Geometry: final body of the model. Coordinates: model frame, mm. A direction names the side the tool comes from. Give positions to 0.01 mm unless a question says otherwise; leave off trailing zeros. Loops run counter-clockwise (first coordinate to the right, second up) from the corner with the lowest first, then second, coordinate; pieces in that order, holes last. Notation, with made-up numbers: (79, 26) -> (134, 26) arc R10 ccw to (134, 34) -> close; hole circle Ø11 at (9, -26.75). An arc over 180 degrees is marked (long way). One line per question, with ' | ' between items. Start each with the question number.
Item 1: Pin query (flat end, axial travel): P1, Ø1.3, axis at y = -23, z = -18.5, coming from the -X side; P2, Ø2, axis at y = -32, z = -20.5, coming from the +X side (3 decimals); P3, Ø2, axis at y = -32, z = -19.5, coming from the -X side (3 decimals). Return the tip coordinate at first contact, or that it passes through.
Item 2: Set-up query: faces 4 (the flat face through (-11, -27.374, -23)), 5 (the flat face through (-3.625, -32, -22)), 6 (the flat face through (-8.705, -32, -22)), 7 (the flat face through (-6, -30.894, -21)), 8 (the cylindrical face through (18.321, 42.327, 1.878)). Return all of +Z, -Z, +X, -X, +Y, -Y with unobstructed straight access to the full face (end or side cutting, diameter ignored); none if empty.
Item 3: Mould query, pull axis Z, two halves, no side actions, for faces 1 (the cylindrical face through (-0.222, -24.665, -6.643)), 2 (the flat face through (0, 0, 0)), 3 (the cylindrical face through (-28.98, -38.59, 1.88)). Classes: released by +Z, released by -Z, zero draft, split by the parting line, or undercut.
Item 4: Section C-C on x = 14. Return loops of the section in (y, z), then the cut area to 3 significant figures.
Item 5: Section D-D on x = 22. Return loops of the section in (y, z).
Item 6: Material intervals for line 1 along Y through (x, z) = (-5, -6.35); line 2 along X through (y, z) = (-21, 2.5) (3 decimals); line 3 along Y through (x, z) = (3, -1), sorted ascending. Write a range as [from, to].
Item 7: Section A-A on y = 40.5. Return loops of the section in (x, z), then the cut area to 3 significant figures.
Item 8: Section B-B on z = -2. Return loops of the section in (x, y) (3 decimals).
from build123d import *

# Parameters (mm, degrees)
BOSS_EXTRUDE2_DEPTH                 = 3.81
BOSS_EXTRUDE4_DEPTH                 = 31.75
F_8_CLEARANCE_HOLE1_D               = 4.4958
PARACHUTE_SHROUD_HOLE_LOW_PROFILE_D = 3.175
MONOFILAMENT_HOLE_LOW_PROFILE_D     = 3.175
BOSS_EXTRUDE7_REACH                 = 67.656
SKETCH21_W                          = 2.032
SKETCH21_H                          = 5.08
SKETCH21_W_2                        = 5.08
SKETCH21_H_2                        = 2.032
SKETCH22_W                          = 11.064
SKETCH22_H                          = 10.632
BOSS_EXTRUDE8_DEPTH                 = 7.894195
BOSS_EXTRUDE9_REACH                 = 87.468
BOSS_EXTRUDE10_DEPTH                = 5.08
FILLET3_R                           = 0.127


with BuildPart() as part:
    # Sketch3 → Boss-Extrude2 (new body)
    with BuildSketch(Plane.XY):
        with BuildLine():
            Line((-15.875, -38.1), (-15.875, 38.1))
            ThreePointArc((-15.875, 38.1), (-18.260491841, 42.291797068), (-23.082694008, 42.38179842))
            ThreePointArc((-23.082694008, 42.38179842), (-28.900226452, 38.649767283), (-34.12497326, 34.12497326))
            ThreePointArc((-34.12497326, 34.12497326), (-35.921024484, 34.12497326), (-35.921024484, 35.921024484))
            ThreePointArc((-35.921024484, 35.921024484), (0, 50.8), (35.921024484, 35.921024484))
            ThreePointArc((35.921024484, 35.921024484), (35.921024484, 34.12497326), (34.12497326, 34.12497326))
            ThreePointArc((34.12497326, 34.12497326), (28.900226452, 38.649767283), (23.082694008, 42.38179842))
            ThreePointArc((23.082694008, 42.38179842), (18.260491841, 42.291797068), (15.875, 38.1))
            Line((15.875, 38.1), (15.875, -38.1))
            ThreePointArc((15.875, -38.1), (18.260491841, -42.291797068), (23.082694008, -42.38179842))
            ThreePointArc((23.082694008, -42.38179842), (28.900226452, -38.649767283), (34.12497326, -34.12497326))
            ThreePointArc((34.12497326, -34.12497326), (35.921024484, -34.12497326), (35.921024484, -35.921024484))
            ThreePointArc((35.921024484, -35.921024484), (0, -50.8), (-35.921024484, -35.921024484))
            ThreePointArc((-35.921024484, -35.921024484), (-35.921024484, -34.12497326), (-34.12497326, -34.12497326))
            ThreePointArc((-34.12497326, -34.12497326), (-28.900226452, -38.649767283), (-23.082694008, -42.38179842))
            ThreePointArc((-23.082694008, -42.38179842), (-18.260491841, -42.291797068), (-15.875, -38.1))
        make_face()
    extrude(amount=BOSS_EXTRUDE2_DEPTH)

    # Sketch5 → Boss-Extrude4 (add)
    with BuildSketch(Plane(origin=(15.875, 0, 0), x_dir=(0, 0, -1), z_dir=(1, 0, 0))):
        with BuildLine():
            Line((0, 38.1), (0, 26.99385))
            Line((0, 26.99385), (0, 14.29385))
            ThreePointArc((0, 14.29385), (1.86498297, 18.77886703), (6.35, 20.64385))
            ThreePointArc((6.35, 20.64385), (12.699998494, 26.998224058), (6.341251887, 33.343843974))
            ThreePointArc((6.341251887, 33.343843974), (2.338844583, 34.612930799), (0, 38.1))
        make_face()
        with BuildLine():
            ThreePointArc((6.261703048, -20.644463916), (1.864650947, -18.840779739), (0, -14.469233029))
            Line((0, -14.469233029), (0, -26.99385))
            Line((0, -26.99385), (0, -38.1))
            ThreePointArc((0, -38.1), (2.217611083, -34.670801888), (6.077775616, -33.338012189))
            ThreePointArc((6.077775616, -33.338012189), (6.213919542, -33.33945129), (6.35, -33.34385))
            ThreePointArc((6.35, -33.34385), (12.7, -26.99385), (6.35, -20.64385))
            ThreePointArc((6.35, -20.64385), (6.305852606, -20.644312569), (6.261703048, -20.644463916))
        make_face()
    extrude(amount=-BOSS_EXTRUDE4_DEPTH)

    # 8 Clearance Hole1 (through all)
    with Locations(Plane(origin=(15.875, 0, 0), x_dir=(0, 0, -1), z_dir=(1, 0, 0))):
        with Locations((6.35, 26.99385), (6.35, -26.893399733)):
            Hole(F_8_CLEARANCE_HOLE1_D / 2)

    # Parachute shroud hole _low profile (through all)
    with Locations(Plane.XY.offset(3.81)):
        with Locations((-9.525, 0)):
            Hole(PARACHUTE_SHROUD_HOLE_LOW_PROFILE_D / 2)

    # Monofilament hole _low profile (through all)
    with Locations(Plane.XY.offset(3.81)):
        with Locations((9.525, 0)):
            Hole(MONOFILAMENT_HOLE_LOW_PROFILE_D / 2)



with BuildPart() as body_2:
    # Boss-Extrude7: up to this plane
    boss_extrude7_end = Plane(origin=(-1.6499976, -20.290855187, -25.429913438), z_dir=(0, 0.01745240643728808, 0.9998476951563912))
    # Sketch21 → Boss-Extrude7 (new, up to the surface)
    with BuildSketch(Plane.XY.offset(-16.509739), mode=Mode.PRIVATE) as boss_extrude7_sk1:
        with BuildLine():
            Line((-2.625, -22.293950072), (-0.593, -22.293950072))
            Line((-0.593, -22.293950072), (-0.593, -27.373950072))
            Line((-0.593, -27.373950072), (-2.625, -27.373950072))
            Line((-2.625, -27.373950072), (-2.625, -25.293950072))
            Line((-2.625, -25.293950072), (-2.575, -25.293950072))
            ThreePointArc((-2.575, -25.293950072), (-2.433578644, -25.235371429), (-2.375, -25.093950072))
            Line((-2.375, -25.093950072), (-2.375, -24.893950072))
            Line((-2.375, -24.893950072), (-2.625, -24.893950072))
            Line((-2.625, -24.893950072), (-2.625, -22.293950072))
        make_face()
    boss_extrude7_tool1 = split(extrude(boss_extrude7_sk1.sketch, amount=-BOSS_EXTRUDE7_REACH, mode=Mode.PRIVATE), bisect_by=boss_extrude7_end, keep=Keep.BOTH, mode=Mode.PRIVATE)
    add(boss_extrude7_tool1.solids().sort_by_distance((-1.600971, -24.831757, -16.509739))[0])
    # Sketch21 → Boss-Extrude7 (new, up to the surface)
    with BuildSketch(Plane.XY.offset(-16.509739), mode=Mode.PRIVATE) as boss_extrude7_sk2:
        with Locations((-10.641, -24.833950072)):
            Rectangle(SKETCH21_W, SKETCH21_H)
    boss_extrude7_tool2 = split(extrude(boss_extrude7_sk2.sketch, amount=-BOSS_EXTRUDE7_REACH, mode=Mode.PRIVATE), bisect_by=boss_extrude7_end, keep=Keep.BOTH, mode=Mode.PRIVATE)
    add(boss_extrude7_tool2.solids().sort_by_distance((-10.641, -24.83395, -16.509739))[0])
    # Sketch21 → Boss-Extrude7 (new, up to the surface)
    with BuildSketch(Plane.XY.offset(-16.509739), mode=Mode.PRIVATE) as boss_extrude7_sk3:
        with Locations((-6.165, -31.909950072)):
            Rectangle(SKETCH21_W_2, SKETCH21_H_2)
    boss_extrude7_tool3 = split(extrude(boss_extrude7_sk3.sketch, amount=-BOSS_EXTRUDE7_REACH, mode=Mode.PRIVATE), bisect_by=boss_extrude7_end, keep=Keep.BOTH, mode=Mode.PRIVATE)
    add(boss_extrude7_tool3.solids().sort_by_distance((-6.165, -31.90995, -16.509739))[0])


with BuildPart() as part_1:
    add(part.part)

    add(body_2.part)  # Boss-Extrude8 merges body 2
    # Sketch22 → Boss-Extrude8 (add)
    with BuildSketch(Plane.XY.offset(-16.509739)):
        with Locations((-6.125, -27.609950072)):
            Rectangle(SKETCH22_W, SKETCH22_H)
    extrude(amount=BOSS_EXTRUDE8_DEPTH)

    # Boss-Extrude9: up to this face of the body (flat: up to its plane)
    boss_extrude9_end = Plane(part_1.part.faces().sort_by_distance((-1.609, -27.373950072, -20.908008278))[0])
    # Sketch23 → Boss-Extrude9 (add, up to the picked face)
    with BuildSketch(Plane(origin=(0, -22.293950072, 0), x_dir=(1, 0, 0), z_dir=(0, 1, 0)), mode=Mode.PRIVATE) as boss_extrude9_sk1:
        Polygon((-11.657, 25.394949287), (-11.657, 28.569949287), (-9.117, 25.394949287), (-9.625, 24.886949287), (-11.657, 24.886949287), align=None)
    boss_extrude9_tool1 = split(extrude(boss_extrude9_sk1.sketch, amount=-BOSS_EXTRUDE9_REACH, mode=Mode.PRIVATE), bisect_by=boss_extrude9_end, keep=Keep.BOTH, mode=Mode.PRIVATE)
    # Sketch23 → Boss-Extrude9 (add, up to the picked face)
    with BuildSketch(Plane(origin=(0, -22.293950072, 0), x_dir=(1, 0, 0), z_dir=(0, 1, 0)), mode=Mode.PRIVATE) as boss_extrude9_sk2:
        Polygon((-0.593, 25.394949287), (-0.593, 28.569949287), (-3.133, 25.394949287), (-2.625, 24.886949287), (-0.593, 24.886949287), align=None)
    boss_extrude9_tool2 = split(extrude(boss_extrude9_sk2.sketch, amount=-BOSS_EXTRUDE9_REACH, mode=Mode.PRIVATE), bisect_by=boss_extrude9_end, keep=Keep.BOTH, mode=Mode.PRIVATE)
    add(boss_extrude9_tool1.solids().sort_by(Axis((-10.743021, -22.29395, -26.161945), (0, -1, 0)))[0])
    add(boss_extrude9_tool2.solids().sort_by(Axis((-1.506979, -22.29395, -26.161945), (0, -1, 0)))[0])

    # Sketch25 → Boss-Extrude10 (add)
    with BuildSketch(Plane(origin=(-3.625, 0, 0), x_dir=(0, 0, -1), z_dir=(1, 0, 0))):
        Polygon((25.209367036, -32.925950072), (28.511367036, -32.925950072), (25.209367036, -30.385950072), (24.701367036, -30.893950072), (24.701367036, -32.925950072), align=None)
    extrude(amount=-BOSS_EXTRUDE10_DEPTH)

    # Fillet3
    fillet3_edges = [part_1.edges().sort_by_distance(p)[0] for p in [
        (-9.117, -24.833950072, -25.394949287),
        (-11.657, -24.833950072, -28.569949287),
        (-0.593, -24.833950072, -28.569949287),
        (-3.133, -24.833950072, -25.394949287),
        (-6.165, -32.925950072, -28.511367036),
        (-6.165, -30.385950072, -25.209367036),
    ]]
    fillet(fillet3_edges, radius=FILLET3_R)


solid = part_1.part
Result sheet:
1) P1: stops at x = -11.66 | P2: stops at x = -3.625 | P3: stops at x = -8.705
2) face 4: -Z, +X, -X, -Y | face 5: -Z, +X, +Y, -Y | face 6: -Z, -X, +Y, -Y | face 7: +X, -X, +Y | face 8: +Z, -Z
3) face 1: undercut | face 2: released by -Z | face 3: zero draft
4) outline: (-48.83, 0) -> (-38.1, 0) arc R6.26 cw to (-33.34, -6.35) arc R6.35 ccw to (-20.64, -6.35) arc R6.26 cw to (-14.47, 0) -> (14.29, 0) arc R6.37 cw to (20.64, -6.35) arc R6.35 ccw to (33.34, -6.34) arc R6.36 cw to (38.1, 0) -> (48.83, 0) -> (48.83, 3.81) -> (-48.83, 3.81) -> close; hole circle Ø4.5 at (-26.89, -6.35); hole circle Ø4.5 at (26.99, -6.35) | area: 660 mm²
5) outline: (-45.79, 0) -> (-42.81, 0) -> (-42.81, 3.81) -> (-45.79, 3.81) -> close; (42.81, 0) -> (45.79, 0) -> (45.79, 3.81) -> (42.81, 3.81) -> close
6) line 1: y = [-33.34, -29.14], [-24.65, -20.64], [20.64, 24.75], [29.24, 33.34] | line 2: x = [-15.875, 15.875] | line 3: y = [-35.94, -17.78], [17.7, 35.98]
7) outline: (-30.67, 0) -> (-26.24, 0) -> (-26.24, 3.81) -> (-30.67, 3.81) -> close; (-16.51, 0) -> (16.51, 0) -> (16.51, 3.81) -> (-16.51, 3.81) -> close; (26.24, 0) -> (30.67, 0) -> (30.67, 3.81) -> (26.24, 3.81) -> close | area: 159 mm²
8) outline: (-15.875, -34.849) -> (15.875, -34.849) -> (15.875, -18.97) -> (-15.875, -18.97) -> close; (-15.875, 18.91) -> (15.875, 18.91) -> (15.875, 34.886) -> (-15.875, 34.886) -> close
